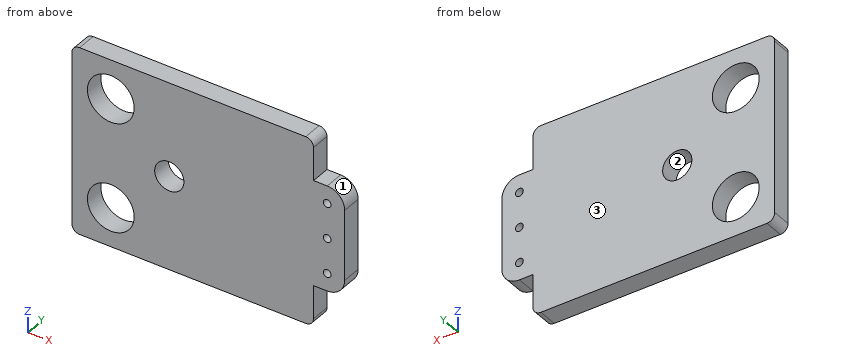
from build123d import *

# Parameters (mm, degrees)
SKETCH1_R           = 6
SKETCH1_R_2         = 3.75
SKETCH1_R_3         = 1
BOSS_EXTRUDE1_DEPTH = 5
FILLET1_R           = 2


with BuildPart() as part:
    # Sketch1 → Boss-Extrude1 (new body)
    with BuildSketch(Plane(origin=(0, 0, 0), x_dir=(1, 0, 0), z_dir=(0, 1, 0))):
        with BuildLine():
            Line((70, 33), (70, 15))
            ThreePointArc((70, 15), (68.681980515, 11.818019485), (65.5, 10.5))
            Line((65.5, 10.5), (62, 10.5))
            Line((62, 10.5), (62, 0))
            Line((62, 0), (0, 0))
            Line((0, 0), (0, 48))
            Line((0, 48), (62, 48))
            Line((62, 48), (62, 37.5))
            Line((62, 37.5), (65.5, 37.5))
            ThreePointArc((65.5, 37.5), (68.681980515, 36.181980515), (70, 33))
        make_face()
        with Locations(Location((10, 10, 0), (0, 0, 270))):
            Circle(SKETCH1_R, mode=Mode.SUBTRACT)
        with Locations(Location((10, 38, 0), (0, 0, 270))):
            Circle(SKETCH1_R, mode=Mode.SUBTRACT)
        with Locations(Location((25, 24, 0), (0, 0, 270))):
            Circle(SKETCH1_R_2, mode=Mode.SUBTRACT)
        with Locations(Location((65.5, 15, 0), (0, 0, 270))):
            Circle(SKETCH1_R_3, mode=Mode.SUBTRACT)
        with Locations(Location((65.5, 24, 0), (0, 0, 270))):
            Circle(SKETCH1_R_3, mode=Mode.SUBTRACT)
        with Locations(Location((65.5, 33, 0), (0, 0, 270))):
            Circle(SKETCH1_R_3, mode=Mode.SUBTRACT)
    extrude(amount=BOSS_EXTRUDE1_DEPTH)

    # Fillet1
    fillet1_edges = [part.edges().sort_by_distance(p)[0] for p in [
        (62, 2.5, 0),
        (0, 2.5, 0),
        (0, 2.5, -48),
        (62, 2.5, -48),
    ]]
    fillet(fillet1_edges, radius=FILLET1_R)


solid = part.part
Source: CAD feature listing. Evaluate the final solid. Frame: model axes, mm. Face numbers are marked on the shaded views. Round coordinates to 2 decimals unless told otherwise and drop trailing zeros. Loops run counter-clockwise (first coordinate to the right, second up) from the corner with the lowest first, then second, coordinate; pieces in that order, holes last.
Q1. Ray query, line 1 (Z direction, x = 65.5, y = 3.5); line 2 (X direction, y = 3.9, z = -10); line 3 (X direction, y = 1.7, z = -33). Return the intervals inside material, ascending.
Q2. Section D-D, the plane z = -35. Return loops of the section in (x, y).
Q3. First-contact query: P1, Ø1, axis at x = 63, y = 3.5, coming from the +Z side; P2, Ø2.5, axis at y = 3, z = -5, coming from the +X side; P3, Ø1.8, axis at x = 64.5, y = 3.5, coming from the -Z side. Flat tips, straight axial feed; report the tip coordinate or a pass-through.
Q4. Section A-A, the plane z = -24. Return loops of the section in (x, y), plus the area to 4 significant figures.
Q5. Section C-C, the plane y = 3.25. Return loops of the section in (x, z).
Q6. Section B-B, the plane x = 10. Return loops of the section in (y, z).
Q7. Mould query, pull axis Z, two halves, no side actions, for the marked faces 1, 2 and 3. Classes: pulls with the +Z half, pulls with the -Z half, needs draft (parallel to the pull), parting line crosses it, or undercut.
Solutions:
1. line 1: z = -37.5 to -34, -32 to -25, -23 to -16, -14 to -10.5
1. line 2: x = 0 to 4, 16 to 62
1. line 3: x = 0 to 6.68, 13.32 to 64.5, 66.5 to 70
2. outline: (0, 0) - (4.8, 0) - (4.8, 5) - (0, 5) - close; (15.2, 0) - (69.53, 0) - (69.53, 5) - (15.2, 5) - close
3. P1: stops at z = -10.5
3. P2: stops at x = 62
3. P3: stops at z = -37.5
4. outline: (0, 0) - (21.25, 0) - (21.25, 5) - (0, 5) - close; (28.75, 0) - (64.5, 0) - (64.5, 5) - (28.75, 5) - close; (66.5, 0) - (70, 0) - (70, 5) - (66.5, 5) - close
4. area: 302.5 mm2
5. outline: (0, -46) arc R2 ccw to (2, -48) - (60, -48) arc R2 ccw to (62, -46) - (62, -37.5) - (65.5, -37.5) arc R4.5 ccw to (70, -33) - (70, -15) arc R4.5 ccw to (65.5, -10.5) - (62, -10.5) - (62, -2) arc R2 ccw to (60, 0) - (2, 0) arc R2 ccw to (0, -2) - close; hole circle Ø12 at (10, -38); hole circle Ø12 at (10, -10); hole circle Ø7.5 at (25, -24); hole circle Ø2 at (65.5, -33); hole circle Ø2 at (65.5, -24); hole circle Ø2 at (65.5, -15)
6. outline: (0, -48) - (5, -48) - (5, -44) - (0, -44) - close; (0, -32) - (5, -32) - (5, -16) - (0, -16) - close; (0, -4) - (5, -4) - (5, 0) - (0, 0) - close
7. face 1: pulls with the +Z half
7. face 2: undercut
7. face 3: needs draft
